Work out the finished part from the listing and answer in its coordinate system (mm). Round coordinates to 2 decimals unless told otherwise and drop trailing zeros. Order: outer loops, then holes, each group sorted by start corner. A loop starts at its lowest first (then second) coordinate and runs counter-clockwise, first axis right, second up. Notation, with made-up numbers: M 9,-6 L 25,-6 A21 ccw 25,9 Z; hole C 76,-3 d10. An arc over 180 degrees is marked long. Return JSON: item names as keys, results as strings.
from build123d import *

# Parameters (mm, degrees)
SKETCH_W                = 190
SKETCH_H                = 132
PAD_DEPTH               = 2.3
SKETCH001_R             = 3.575
POCKET_DEPTH            = 465.028955
SKETCH001_MIRRORED_2_R  = 3.575
POCKET_MIRRORED_2_DEPTH = 465.028955
LINEARPATTERN_COUNT     = 2
LINEARPATTERN_PITCH     = 116.5


with BuildPart() as part:
    # Sketch → Pad (new body)
    with BuildSketch(Plane.XY):
        Rectangle(SKETCH_W, SKETCH_H)
    extrude(amount=PAD_DEPTH)

    # Sketch001 (on Face6 of Pad) → Pocket (cut, through all)
    with BuildSketch(Plane.XY.offset(2.3)):
        with Locations((-89.9, 57.5)):
            Circle(SKETCH001_R)
    pocket = extrude(amount=-POCKET_DEPTH, mode=Mode.SUBTRACT)

    # Sketch001 Mirrored 2 → Pocket Mirrored 2 (cut, through all)
    with BuildSketch(Plane(origin=(0, 0, 2.3), x_dir=(-1, 0, 0), z_dir=(0, 0, -1))):
        with Locations((-89.9, 57.5)):
            Circle(SKETCH001_MIRRORED_2_R)
    pocket_mirrored_2 = extrude(amount=POCKET_MIRRORED_2_DEPTH, mode=Mode.SUBTRACT)

    # LinearPattern: Pocket, Pocket Mirrored 2 ×2
    with Locations(*[(0, -i * LINEARPATTERN_PITCH, 0) for i in range(1, LINEARPATTERN_COUNT)]):
        add(pocket, mode=Mode.SUBTRACT)
        add(pocket_mirrored_2, mode=Mode.SUBTRACT)


solid = part.part
Item 1: The mould has two halves that part along X. Classify faces 1 (the cylindrical face through (-93.47, 57.66, 1.17)), 2 (the flat face through (-1, 1, 2.3)): pulls with the +X half, pulls with the -X half, needs draft (parallel to the pull), parting line crosses it, or undercut.
Output:
{"face 1": "undercut", "face 2": "needs draft"}
Item 2: Consider line 1 along Y through (x, z) = (-89.9, 1.4) (3 decimals). Determine where the line is inside the solid, lowest interval first. Write a range as [from, to].
Output:
{"line 1": "y = [-66, -62.575], [-55.425, 53.925], [61.075, 66]"}
Item 3: This flat-tipped pin is pushed along its axis until it touches: pin 1 (5.5 mm diameter, centred on x = 89.9, y = -59, fed in from -Z). Where does it stop, or does it pass through?
Output:
{"pin 1": "passes through"}
Item 4: Find section B-B (x = 89.9). Determine the outline of the cut face in (y, z) (3 decimals), plus the area to 3 significant figures.
Output:
{"outline": "M -66,0 L -62.575,0 L -62.575,2.3 L -66,2.3 Z; M -55.425,0 L 53.925,0 L 53.925,2.3 L -55.425,2.3 Z; M 61.075,0 L 66,0 L 66,2.3 L 61.075,2.3 Z", "area": "271 mm^2"}
Item 5: Find section A-A (y = -59). Determine the outline of the cut face in (x, z) (3 decimals).
Output:
{"outline": "M -95,0 L -93.475,0 L -93.475,2.3 L -95,2.3 Z; M -86.325,0 L 86.325,0 L 86.325,2.3 L -86.325,2.3 Z; M 93.475,0 L 95,0 L 95,2.3 L 93.475,2.3 Z"}
